Read the model definition and answer for the solid it produces. Units are mm, in the model's axes. Round coordinates to 2 decimals unless told otherwise and drop trailing zeros. Loops run counter-clockwise (first coordinate to the right, second up) from the corner with the lowest first, then second, coordinate; pieces in that order, holes last. Notation, with made-up numbers: M 15,33 L 60,33 A21 cw 60,40 Z; hole C 19.5,56.5 d11. An arc over 180 degrees is marked long. Write each question's results on one line, items separated by ' | '.
```python
from build123d import *

# Parameters (mm, degrees)
SKETCH1_W              = 4.318
SKETCH1_H              = 84.836
BOSS_EXTRUDE1_DEPTH    = 3.556
CUT_EXTRUDE2_START     = -1.583272769
CUT_EXTRUDE2_OUTLINE_W = 2.54
CUT_EXTRUDE2_OUTLINE_H = 2.032
CUT_EXTRUDE2_DEPTH     = 1.583272769


# Read off the part's stored shape, not the designer's step: Cut-Extrude2
with BuildPart() as part:
    # Sketch1 → Boss-Extrude1 (new body)
    with BuildSketch(Plane(origin=(0, 0, 0), x_dir=(1, 0, 0), z_dir=(0, 1, 0))):
        with Locations((-65.659, 42.418)):
            Rectangle(SKETCH1_W, SKETCH1_H)
    extrude(amount=BOSS_EXTRUDE1_DEPTH)

    # Cut-Extrude2 outline → Cut-Extrude2 (cut)
    with BuildSketch(Plane(origin=(-63.5, 0, 0), x_dir=(0, 0, -1), z_dir=(1, 0, 0)).offset(CUT_EXTRUDE2_START)):
        with Locations((42.418, 2.54)):
            Rectangle(CUT_EXTRUDE2_OUTLINE_W, CUT_EXTRUDE2_OUTLINE_H)
    extrude(amount=CUT_EXTRUDE2_DEPTH, mode=Mode.SUBTRACT)


solid = part.part
```
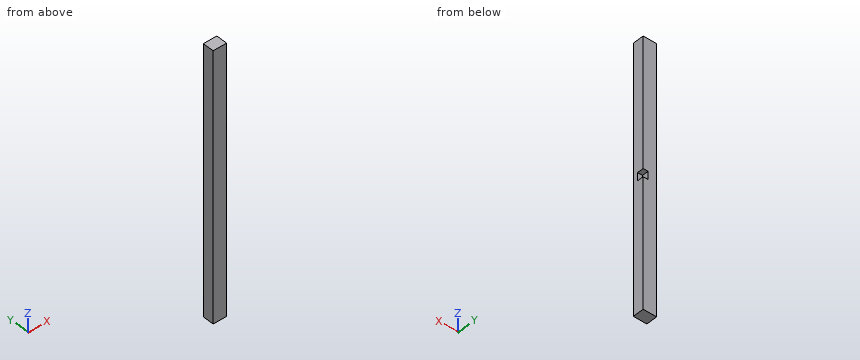
1. Given P1, Ø1.3, axis at x = -64, z = -42.5, coming from the +Y side, flat-ended and moving along its own axis, determine where the tip first touches the part or whether it passes through.
Completed:
P1: stops at y = 1.52
2. Find the intervals of material crossed by L1, parallel to Z at x = -63.75, y = 2.65; L2, parallel to X at y = 3.1, z = -43.5, in increasing order.
Completed:
L1: z = -84.84 to -43.69, -41.15 to 0 | L2: x = -67.82 to -65.08
3. Find section A-A, the plane x = -64.15. Give the vertices of the cut face in (y, z), then the cut area to 3 significant figures.
Completed:
outline: M 0,-84.84 L 3.56,-84.84 L 3.56,-43.69 L 1.52,-43.69 L 1.52,-41.15 L 3.56,-41.15 L 3.56,0 L 0,0 Z | area: 297 mm2
